Build history of the part. All positions in model axes, mm. Face numbers are marked on the shaded views. A direction names the side the tool comes from. Coordinates: 2 decimals unless noted, no trailing zeros. Loops run counter-clockwise (first coordinate to the right, second up) from the corner with the lowest first, then second, coordinate; pieces in that order, holes last.
Item 1: Drill centre lines: line 1 along X through (y, z) = (-0.4, 2); line 2 along X through (y, z) = (-0.2, 1.4); line 3 along Y through (x, z) = (-2, 0.7). Where is each one in solid material? Low to high.
Item 2: Cut at B-B (x = 2.75). List the corners of the cut face in (y, z), and give its area (3 significant figures).
Item 3: 3-axis set-ups, long thin cutter, end or side, ignore diameter. For the marked faces 1 and 2: which of +Z, -Z, +X, -X, +Y, -Y reach the whole face in a straight line?
Item 4: Flat gauge pins, fed straight in: pin 1 (1.5 mm diameter, centred on x = -1, z = -2, fed in from -Y); pin 2 (1 mm diameter, centred on x = -1.5, z = -2, fed in from +Y); pin 3 (3 mm diameter, centred on y = 1, z = -1, fed in from +X); pin 4 (1 mm diameter, centred on x = 1, z = 1, fed in from -Y). Where does each tip first touch, or does it go through?
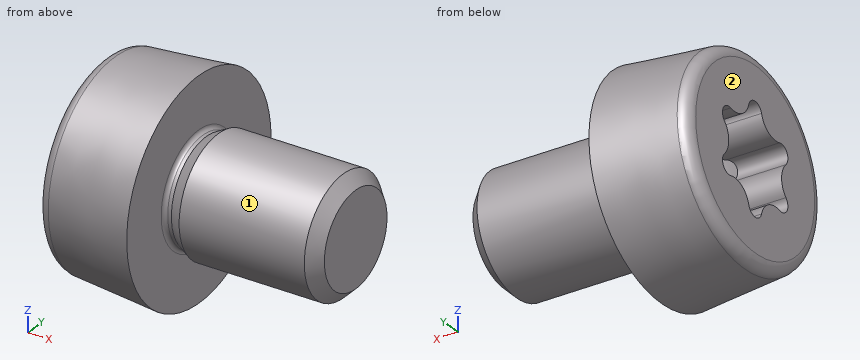
Autodesk Inventor part; units mm, degrees
ref_plane "Work Plane1" through (0, 0, 0) normal (0, 0.5, 0.866) x (1, 0, 0)
ref_plane "YZ Plane" through (0, 0, 0) normal (1, 0, 0) x (0, 1, 0)
ref_plane "XZ Plane" through (0, 0, 0) normal (0, 1, 0) x (-1, 0, 0)
sketch "Sketch1" plane through (0, 0, 0) normal (0, 0, 1) x (1, 0, 0)
  line L0 (-0.3217, 0) -> (4, 0)
  line L1 (4, 0) -> (4, 1.5)
  line L2 (4, 1.5) -> (0.5, 1.5)
  line L3 (0.5, 1.5) -> (0.1933, 1.3375)
  line L4 (0.1933, 1.3375) -> (0.1, 1.3375)
  line L5 (0, 1.4375) -> (0, 2.75)
  line L6 (0, 2.75) -> (-2.4, 2.75)
  line L7 (-2.4, 2.75) -> (-2.4, 1.4)
  line L8 (-2.4, 1.4) -> (-1.13, 1.4)
  line L9 (-1.13, 1.4) -> (-0.3217, 0)
  line L10 (-3.68, 0) -> (5.28, 0)
  line L11 (0, -0.55) -> (0, 3.3)
  line L12 (0.5, 1.5) -> (0, 1.5) construction
  arc A0 (0, 1.4375) -> (0.1, 1.3375) centre (0.1, 1.4375) ccw
  line L13 (0, 2.75) -> (-2.4, 2.54)
  point P0 (0, 1.3375)
  dimension "d1" = 3.5
  dimension "d2" = 0.3067
  dimension "d3" = 2.4
  dimension "d4" = 1.27
  dimension "d5" = 60
  dimension "d6" = 3
  dimension "d7" = 2.675
  dimension "d8" = 2.8
  dimension "d9" = 5.5
  dimension "d20" = 4
  dimension "d34" = 0.1
  dimension "d35" = 5
revolve "Body" add sketch "Sketch1" angle 360 about axis through (-0.3217, 0, 0) along (1, 0, 0)
sketch "Sketch2" plane through (-2.4, 0, 0) normal (-1, 0, 0) x (0, 0, 1)
  line L0 (0, -4.9779) -> (0, 10.6176)
  line L1 (-5.0424, 0) -> (11.0045, 0)
  circle A0 centre (0, 0) radius 2.75
  circle A1 centre (0, 0) radius 1.0072
  line L2 (0, 0) -> (4.8438, 8.3897) construction
  line L3 (0, 0) -> (8.7121, 5.0299) construction
  circle A2 centre (0, 0) radius 1.4
  arc A3 (0.8164, 0.9308) -> (0.3979, 1.1724) centre (0.575, 0.9959) ccw
  arc A4 (1.2143, -0.2416) -> (1.2143, 0.2416) centre (1.15, 0) ccw
  arc A5 (0.8164, 0.9308) -> (1.2143, 0.2416) centre (1.3588, 0.7845) ccw
  arc A6 (-0.3979, 1.1724) -> (-0.8164, 0.9308) centre (-0.575, 0.9959) ccw
  arc A7 (-1.2143, 0.2416) -> (-1.2143, -0.2416) centre (-1.15, 0) ccw
  arc A8 (-1.2143, 0.2416) -> (-0.8164, 0.9308) centre (-1.3588, 0.7845) ccw
  arc A9 (0.3979, -1.1724) -> (0.8164, -0.9308) centre (0.575, -0.9959) ccw
  arc A10 (1.2143, -0.2416) -> (1.2143, 0.2416) centre (1.15, 0) ccw
  arc A11 (1.2143, -0.2416) -> (0.8164, -0.9308) centre (1.3588, -0.7845) ccw
  arc A12 (-0.8164, -0.9308) -> (-0.3979, -1.1724) centre (-0.575, -0.9959) ccw
  arc A13 (-0.8164, -0.9308) -> (-1.2143, -0.2416) centre (-1.3588, -0.7845) ccw
  arc A14 (-1.2143, 0.2416) -> (-1.2143, -0.2416) centre (-1.15, 0) ccw
  arc A15 (-0.3979, 1.1724) -> (0.3979, 1.1724) centre (0, 1.569) ccw
  arc A16 (0.3979, -1.1724) -> (-0.3979, -1.1724) centre (0, -1.569) ccw
  dimension "d38" = 2.0144
  dimension "d39" = 30
  dimension "d40" = 60
  dimension "d42" = 0.25
extrude "Slot" add sketch "Sketch2" against normal up to next contours A2 A12 A16 L0 | L0 A16 A9 A2 | A2 A7 A13 A12 | A9 A11 A4 A2 | A2 A6 A8 A7 | A4 A5 A3 A2 | A2 L0 A15 A6 | A2 A3 A15 L0
revolve "Taper" cut sketch "Sketch1" angle 360 about axis through (0, 0, 0) along (1, 0, 0) contours L13 L7 L6
fillet "Fillet1" radius 0.3 1 edges at (-2.4, -2.54, 0)
thread "Thread"
chamfer "Chamfer1" distance 0.3067 distance2 0.3068 1 edges at (4, -1.5, 0) measured on face at (4, -0.2617, -0.7882)
ref_plane "Work Plane1" through (0, 0, 0) normal (0, 0.5, 0.866) x (1, 0, 0)
equation "\"d1\" = GEL"
equation "\"d2\" = GAL"
equation "\"d3\" = KOH"
equation "\"d4\" = INTI"
equation "\"d6\" = GD"
equation "\"d7\" = BDM"
equation "\"d8\" = E0"
equation "\"d9\" = KOD"
equation "\"d20\" = NLG"
equation "\"d34\" = R"
equation "\"d38\" = SW"
equation "\"d42\" = RRK"
equation "\"d17\" = RR"
equation "\"d13\" = GEL"
equation "\"d15\" = -0.5 * SPD + 0.5 * GD"
equation "\"GD\" = NND"
equation "\"NLG\" = 4"
equation "\"GEL\" = 3.5"
equation "\"KOD\" = 5.5"
equation "\"KOH\" = 2.4"
equation "\"INTI\" = 1.27"
equation "\"GAL\" = 0.61345 * PTC"
equation "\"GUL\" = 0.61345 * PTC"
equation "\"BDM\" = 2.675"
equation "\"SW\" = 2.0144"
equation "\"RR\" = 0.3"
equation "\"SPD\" = NND - 1.2269 * PTC"
equation "\"R\" = 0.1"
equation "\"E0\" = 2.8"
equation "\"RRK\" = 0.25"
equation "\"PHH\" = 0"
equation "\"GD1\" = THREADDIA - 1.2269 * PTC"
equation "\"THREADDIA\" = 3"
equation "\"FAWI\" = 90deg"
equation "\"ANG\" = 120deg"
equation "\"PTC\" = 0.5"
equation "\"NND\" = 3"
equation "\"TOA\" = 30deg"
equation "\"KEWI\" = 5deg"
properties part number "Screw GB/T 2171.1 M3 x 4" material "Steel, Mild"
Filled sheet:
1. line 1: x = -2.4 to 0
1. line 2: x = -2.4 to 0, 0.34 to 3.78
1. line 3: y = -2.48 to -1.21, 1.21 to 2.48
2. outline: circle Ø3 at (0, 0)
2. area: 7.07 mm2
3. face 1: +X
3. face 2: +Z, -Z, -X, +Y, -Y
4. pin 1: stops at y = -2.36
4. pin 2: stops at y = 2.15
4. pin 3: stops at x = 4
4. pin 4: stops at y = -1.41
